Input: dimensioned drawing with shaded views. Units: mm. Origin: part minimum x, y, z. A direction names the side the tool comes from. Give positions to 0.01 mm unless a question says otherwise; leave off trailing zeros. Loops run counter-clockwise (first coordinate to the right, second up) from the corner with the lowest first, then second, coordinate; pieces in that order, holes last. Notation, with made-up numbers: M -27.75,59 L 28.25,59 A10 ccw 28.25,77 Z; hole C 18.25,38 d2. An arc over 180 degrees is marked long. Answer in a Markdown table with one row per item.
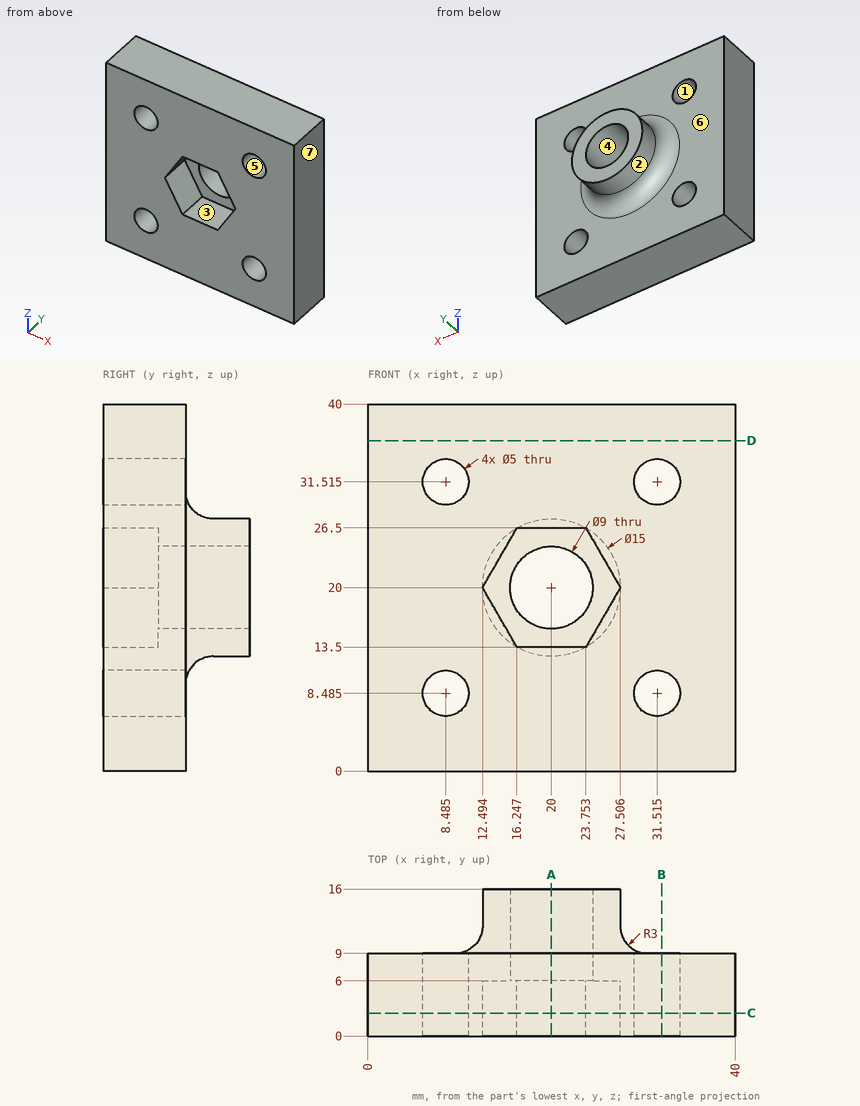
Q1. Section query C-C (y = 2.5). Output: boundary loops of the cut face in (x, z) (1 decimal), plus the area to 4 significant figures.
Values follow:
| item | result |
|---|---|
| outline | M 0,0 L 40,0 L 40,40 L 0,40 Z; hole C 8.5,8.5 d5; hole C 8.5,31.5 d5; hole M 12.5,20 L 16.2,13.5 L 23.8,13.5 L 27.5,20 L 23.8,26.5 L 16.2,26.5 Z; hole C 31.5,8.5 d5; hole C 31.5,31.5 d5 |
| area | 1,375 mm^2 |
Q2. Section query A-A (x = 20). Output: boundary loops of the cut face in (y, z).
Values follow:
| item | result |
|---|---|
| outline | M 0,0 L 9,0 L 9,9.5 A3 cw 12,12.5 L 16,12.5 L 16,15.5 L 6,15.5 L 6,13.5 L 0,13.5 Z; M 0,26.5 L 6,26.5 L 6,24.5 L 16,24.5 L 16,27.5 L 12,27.5 A3 cw 9,30.5 L 9,40 L 0,40 Z |
Q3. Reachability of the marked faces 1, 2 and 3 from +Z, -Z, +X, -X, +Y, -Y: full face, straight path, thin tool, end or side. Return the list, or none.
Values follow:
| item | result |
|---|---|
| face 1 | +Y, -Y |
| face 2 | +Y |
| face 3 | -Y |
Q4. Contact query for flat-ended pins moving along their axis: pin 1 Ø6 at (x, y) = (34, 13) entering from -Z; pin 2 Ø3 at (x, z) = (4.5, 15.5) entering from +Y; pin 3 Ø1.5 at (x, y) = (13, 11.5) entering from -Z (1 decimal). Output: stop coordinate, or through.
Values follow:
| item | result |
|---|---|
| pin 1 | through |
| pin 2 | y = 9 |
| pin 3 | z = 15.7 |
Q5. Section query B-B (x = 32). Output: boundary loops of the cut face in (y, z), plus the area to 3 significant figures.
Values follow:
| item | result |
|---|---|
| outline | M 0,0 L 9,0 L 9,6.03 L 0,6.03 Z; M 0,10.94 L 9,10.94 L 9,29.06 L 0,29.06 Z; M 0,33.97 L 9,33.97 L 9,40 L 0,40 Z |
| area | 272 mm^2 |
Q6. Section query D-D (z = 36). Output: boundary loops of the cut face in (x, y).
Values follow:
| item | result |
|---|---|
| outline | M 0,0 L 40,0 L 40,9 L 0,9 Z |
Q7. Ray query, probe 1 along X at (y, z) = (8.75, 31.5) (1 decimal); probe 2 along X at (y, z) = (8.25, 30.5); probe 3 along Z at (x, y) = (33.5, 7.5) (1 decimal). Return the intervals inside material, ascending. Write a range as from..to.
Values follow:
| item | result |
|---|---|
| probe 1 | 0..6, 11..29, 34..40 |
| probe 2 | 0..6.2, 10.77..29.23, 33.8..40 |
| probe 3 | 0..7, 10..30, 33..40 |
Q8. Mould query, pull axis X, two halves, no side actions, for the marked faces 4, 5, 6 and 7. Classes: +X half, -X half, draft (parallel to the pull), parting line (faces both ways), or undercut.
Values follow:
| item | result |
|---|---|
| face 4 | undercut |
| face 5 | undercut |
| face 6 | draft |
| face 7 | +X half |
